Autodesk Inventor part; units mm, degrees
ref_plane "YZ Plane" through (0, 0, 0) normal (1, 0, 0) x (0, 1, 0)
ref_plane "XZ Plane" through (0, 0, 0) normal (0, 1, 0) x (-1, 0, 0)
ref_plane "XY Plane" through (0, 0, 0) normal (0, 0, 1) x (1, 0, 0)
sketch "Sketch1" plane through (0, 0, 0) normal (1, 0, 0) x (0, 1, 0)
  circle A0 centre (0, 0) radius 2.54
  arc A1 (0, -9.525) -> (0, 9.525) centre (0, 0) ccw
  line L0 (0, 9.525) -> (-101.6, 9.525)
  line L1 (-101.6, -9.525) -> (0, -9.525)
  arc A2 (-49.53, -2.54) -> (-49.53, 2.54) centre (-49.53, 0) ccw
  line L2 (-49.53, 2.54) -> (-101.6, 2.54)
  line L3 (-49.53, -2.54) -> (-101.6, -2.54)
  arc A3 (-101.6, 2.54) -> (-101.6, -2.54) centre (-101.6, 0) ccw
  arc A4 (-101.6, 9.525) -> (-101.6, -9.525) centre (-101.6, 0) ccw
  point P0 (-111.76, 0)
  dimension "d0" = 5.08
  dimension "d12" = 5.08
  dimension "d17" = 52.07
extrude "Extrusion1" add sketch "Sketch1" along normal blind 1.5875
properties part number "hgsupport"
Source: CAD feature listing. Evaluate the final solid. Frame: model axes, mm. A direction names the side the tool comes from. Coordinates: 2 decimals unless noted, no trailing zeros. Loops run counter-clockwise (first coordinate to the right, second up) from the corner with the lowest first, then second, coordinate; pieces in that order, holes last. Notation, with made-up numbers: (12.5, 63) -> (69.5, 63) arc R13 ccw to (69.5, 73) -> close; hole circle Ø3 at (56.5, -28). An arc over 180 degrees is marked (long way). Answer in a Markdown table with one row per item. Add a question column.
Q1. Reachability of faces 1 (the face through (0.783, -111.123, -0.209)), 2 (the face through (0.78, -104.14, -0.06)) from +Z, -Z, +X, -X, +Y, -Y: full face, straight path, thin tool, end or side. Return the list, or none.
Q2. Section A-A on y = -91. Return the cut outline in (x, z) (1 decimal), and give its area (3 significant figures).
Q3. Ray query, line 1 along Z through (x, y) = (0.4, -78.5) (3 decimals); line 2 along Y through (x, z) = (0.85, 1.75); line 3 along Y through (x, z) = (0.85, -2). Return the intervals inside material, ascending.
Q4. Contact query for a flat-ended pin moving along its axis: pin 1 Ø6 at (y, z) = (-60, -1) entering from +X. Output: stop coordinate, or through.
Q5. Section C-C on x = 1.2. Return the cut outline in (y, z) (3 decimals).
Q6. Pull-direction query (Z, two-part tool) for faces 3 (the face through (1.588, -52, 4)), 4 (the face through (0.783, 9.523, 0.209)), 5 (the face through (0.78, -46.99, 0.06)); classes: pulls with the +Z half, pulls with the -Z half, needs draft (parallel to the pull), parting line crosses it, or undercut.
Q7. Section D-D on y = -1.5. Return the cut outline in (x, z) (1 decimal), and give its area (3 significant figures).
Q8. Section B-B on z = 0. Return the cut outline in (x, y) (1 decimal).
Computed values:
| question | item | result |
|---|---|---|
| 1 | face 1 | +X, -X, -Y |
| 1 | face 2 | +X, -X |
| 2 | outline | (0, -9.5) -> (1.6, -9.5) -> (1.6, -2.5) -> (0, -2.5) -> close; (0, 2.5) -> (1.6, 2.5) -> (1.6, 9.5) -> (0, 9.5) -> close |
| 2 | area | 22.2 mm^2 |
| 3 | line 1 | z = -9.525 to -2.54, 2.54 to 9.525 |
| 3 | line 2 | y = -110.96 to -103.44, -47.69 to -1.84, 1.84 to 9.36 |
| 3 | line 3 | y = -110.91 to -103.17, -47.96 to -1.57, 1.57 to 9.31 |
| 4 | pin 1 | stops at x = 1.59 |
| 5 | outline | (-101.6, -9.525) -> (0, -9.525) arc R9.525 ccw to (0, 9.525) -> (-101.6, 9.525) arc R9.525 ccw to start; hole (-101.6, -2.54) -> (-49.53, -2.54) arc R2.54 ccw to (-49.53, 2.54) -> (-101.6, 2.54) arc R2.54 ccw to start; hole circle Ø5.08 at (0, 0) |
| 6 | face 3 | needs draft |
| 6 | face 4 | parting line crosses it |
| 6 | face 5 | undercut |
| 7 | outline | (0, -9.5) -> (1.6, -9.5) -> (1.6, -2) -> (0, -2) -> close; (0, 2) -> (1.6, 2) -> (1.6, 9.5) -> (0, 9.5) -> close |
| 7 | area | 23.7 mm^2 |
| 8 | outline | (0, -111.1) -> (1.6, -111.1) -> (1.6, -104.1) -> (0, -104.1) -> close; (0, -47) -> (1.6, -47) -> (1.6, -2.5) -> (0, -2.5) -> close; (0, 2.5) -> (1.6, 2.5) -> (1.6, 9.5) -> (0, 9.5) -> close |
